Work out the finished part from the listing and answer in its coordinate system (mm). Face numbers are marked on the shaded views. A direction names the side the tool comes from. Give positions to 0.01 mm unless a question says otherwise; leave off trailing zeros. Order: outer loops, then holes, each group sorted by start corner. A loop starts at its lowest first (then second) coordinate and runs counter-clockwise, first axis right, second up. Notation, with made-up numbers: (62, 81) - (81, 81) arc R6 cw to (81, 88) - close; hole circle Ø5 at (42.25, 41). An arc over 180 degrees is marked (long way). Return JSON: item names as keys, results as strings. Group by question number.
from build123d import *

# Parameters (mm, degrees)
SKETCH_W     = 25
SKETCH_H     = 13
SKETCH_R     = 4.5
PAD_DEPTH    = 20
POCKET_DEPTH = 12.4


with BuildPart() as part:
    # Sketch → Pad (new body)
    with BuildSketch(Plane.XY):
        Rectangle(SKETCH_W, SKETCH_H)
        Circle(SKETCH_R, mode=Mode.SUBTRACT)
    extrude(amount=PAD_DEPTH)

    # Sketch001 → Pocket (cut)
    with BuildSketch(Plane.XY.offset(20)):
        Polygon((-7.505554, 0), (-3.752777, -6.5), (3.752777, -6.5), (7.505554, 0), (3.752777, 6.5), (-3.752777, 6.5), align=None)
    extrude(amount=-POCKET_DEPTH, mode=Mode.SUBTRACT)


solid = part.part
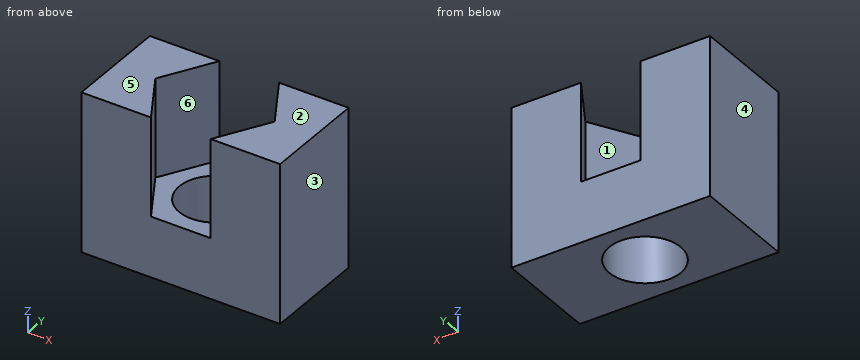
1. Consider probe 1 along X at (y, z) = (0, 2.5); probe 2 along X at (y, z) = (1.75, 8); probe 3 along Y at (x, z) = (0, 5). Determine where each line is inside the solid, lowest interval first. Write a range as from..to.
2. A tool of negligible diameter and unlimited length cuts with its end or side. For the marked faces 5 and 6, from which of +Z, -Z, +X, -X, +Y, -Y can it reach the whole face along a straight path? Write none if from no direction.
3. The part is cut by section D-D (y = -1.25). Give the vertices of the cut face in (x, z), and give its area (3 significant figures).
4. Determine the mould class of the marked faces 1, 2, 3 and 4 for opening direction X: released by +X, released by -X, zero draft, split by the parting line, or undercut.
5. The part is cut by section B-B (x = 0). Give the vertices of the cut face in (y, z).
6. The part is cut by section A-A (z = 10.5). Give the vertices of the cut face in (x, y).
7. The part is cut by section C-C (z = 7). Give the vertices of the cut face in (x, y).
Answers:
{
 "1": {"probe 1": "x = -12.5..-4.5, 4.5..12.5", "probe 2": "x = -12.5..-6.5, 6.5..12.5", "probe 3": "y = -6.5..-4.5, 4.5..6.5"},
 "2": {"face 5": "+Z, +X, -X, +Y, -Y", "face 6": "+Z"},
 "3": {"outline": "(-12.5, 0) - (-4.32, 0) - (-4.32, 7.6) - (-6.78, 7.6) - (-6.78, 20) - (-12.5, 20) - close; (4.32, 0) - (12.5, 0) - (12.5, 20) - (6.78, 20) - (6.78, 7.6) - (4.32, 7.6) - close", "area": "266 mm^2"},
 "4": {"face 1": "undercut", "face 2": "zero draft", "face 3": "released by +X", "face 4": "released by -X"},
 "5": {"outline": "(-6.5, 0) - (-4.5, 0) - (-4.5, 7.6) - (-6.5, 7.6) - close; (4.5, 0) - (6.5, 0) - (6.5, 7.6) - (4.5, 7.6) - close"},
 "6": {"outline": "(-12.5, -6.5) - (-3.75, -6.5) - (-7.51, 0) - (-3.75, 6.5) - (-12.5, 6.5) - close; (3.75, -6.5) - (12.5, -6.5) - (12.5, 6.5) - (3.75, 6.5) - (7.51, 0) - close"},
 "7": {"outline": "(-12.5, -6.5) - (12.5, -6.5) - (12.5, 6.5) - (-12.5, 6.5) - close; hole circle Ø9 at (0, 0)"}
}
